Read the model definition and answer for the solid it produces. Units are mm, in the model's axes. A direction names the side the tool comes from. Coordinates: 2 decimals unless noted, no trailing zeros. Write each loop counter-clockwise with the first axis right and the second up, starting at its lowest first coordinate (ties: lowest second). Pieces come first, ordered by that corner, then holes. Notation, with made-up numbers: (51, -11) -> (62, -11) arc R22 cw to (62, 16) -> close; hole circle Ø6 at (-13.75, 65). An arc over 180 degrees is marked (long way). Answer as a JSON object with one key per item and string values. Group by question number.
(1) Find section A-A (y = -10). Give the vertices of the cut face in (x, z), then the cut area to 3 significant figures.
(2) Find section B-B (x = -7.5). Give the vertices of the cut face in (y, z).
(3) Straight lines are drawn through the part: L1, parallel to X at y = 13.14, z = -3.6; L2, parallel to Y at x = 13.25, z = -0.3; L3, parallel to X at y = 23.8, z = -2.5. For each, find the intervals that lie inside material, in ascending order.
(4) Which of the six approach directions +Z, -Z, +X, -X, +Y, -Y give full straight-line access (tool end or side, diameter ignored) to faces 4 (the face through (6, -29, -2)), 5 (the face through (-12.695, -24.458, -2.138)), 6 (the face through (-13, 27.5, -2)), 7 (the face through (-6, -29, -2)), 8 (the face through (11, 27.5, -2))?
(5) For a pull along Z with two mould halves and no side action, classify faces 1 (the face through (0, -13, 0)), 2 (the face through (-12, -21.5, -2)), 3 (the face through (13.106, -12.357, -2.535)) as +Z half, -Z half, draft (parallel to the pull), parting line (faces both ways), or undercut.
(6) Flat-ended cylindrical pins translate along their axes: P1, Ø1.3, axis at x = 12, z = -2, coming from the -Y side; P2, Ø1.7, axis at x = -12, z = -2.5, coming from the +Y side. Find the tip coordinate at first contact, or state that the pin passes through.
(7) Find section C-C (z = -0.75). Give the vertices of the cut face in (x, y).
Autodesk Inventor part; units mm, degrees
ref_plane "YZ Plane" through (0, 0, 0) normal (1, 0, 0) x (0, 1, 0)
ref_plane "XZ Plane" through (0, 0, 0) normal (0, 1, 0) x (-1, 0, 0)
ref_plane "XY Plane" through (0, 0, 0) normal (0, 0, 1) x (1, 0, 0)
sketch "Sketch1" plane through (0, 0, 0) normal (0, 0, 1) x (1, 0, 0)
  line L0 (15, 27.5) -> (-15, 27.5)
  line L1 (-15, 27.5) -> (-15, -27.5)
  line L2 (-15, -27.5) -> (15, -27.5)
  line L3 (15, -27.5) -> (15, 27.5)
  line L4 (15, 27.5) -> (-15, -27.5) construction
  line L5 (-15, 27.5) -> (15, -27.5) construction
  line L6 (13.14, 13.14) -> (-13.14, 13.14) construction
  line L7 (-13.14, 13.14) -> (-13.14, -13.14) construction
  line L8 (-13.14, -13.14) -> (13.14, -13.14) construction
  line L9 (13.14, -13.14) -> (13.14, 13.14) construction
  line L10 (13.14, 13.14) -> (-13.14, -13.14) construction
  line L11 (-13.14, 13.14) -> (13.14, -13.14) construction
  line L12 (15, 15) -> (-15, 15) construction
  line L13 (-15, 15) -> (-15, -15) construction
  line L14 (-15, -15) -> (15, -15) construction
  line L15 (15, -15) -> (15, 15) construction
  line L16 (15, 15) -> (-15, -15) construction
  line L17 (-15, 15) -> (15, -15) construction
  line L18 (0, 27.5) -> (0, -27.5) construction
  line L19 (15, 0) -> (-15, 0) construction
  line L20 (6, 27.5) -> (6, 30.5)
  line L21 (6, 30.5) -> (-6, 30.5)
  line L22 (-6, 30.5) -> (-6, 27.5)
  arc A0 (-9, 27.5) -> (-6, 27.5) centre (-7.5, 27.5) ccw
  line L23 (-15.1, -15.1) -> (15.1, 15.1) construction
  line L24 (15.1, -15.1) -> (-15.1, 15.1) construction
  line L25 (6, -27.5) -> (6, -30.5)
  line L26 (6, -30.5) -> (-6, -30.5)
  line L27 (-6, -30.5) -> (-6, -27.5)
  arc A1 (-6, -27.5) -> (-9, -27.5) centre (-7.5, -27.5) ccw
  line L28 (-12, 27.5) -> (-12, 21.5) construction
  line L29 (0, 30.5) -> (0, 27.5) construction
  line L30 (12, 27.5) -> (12, 21.5) construction
  arc A2 (6, 27.5) -> (9, 27.5) centre (7.5, 27.5) ccw
  line L31 (12, -27.5) -> (12, -21.5) construction
  arc A3 (9, -27.5) -> (6, -27.5) centre (7.5, -27.5) ccw
  circle A4 centre (0, 0) radius 12.5
  point P0 (13.14, -13.14)
  point P1 (-9, -27.5)
  point P2 (6, 28)
  point P3 (6, -27.5)
  point P4 (-6, -27.5)
  point P5 (-6, -27.5)
  point P6 (6, -27.5)
  point P7 (9, -27.5)
  dimension "d0" = 26.28
  dimension "d1" = 26.28
  dimension "d2" = 30
  dimension "d3" = 30
  dimension "d19" = 3
  dimension "d20" = 12
  dimension "d37" = 55
  dimension "d40" = 6
  dimension "d41" = 6
  dimension "d50" = 12.5
  dimension "d57" = 30
  dimension "d60" = 1.5
  dimension "d62" = 25
extrude "Extrusion1" add sketch "Sketch1" against normal blind 5 contours L3 L2 A3 A1 L1 L0 A0 A2 | L0 L22 L21 L20 | L25 L26 L27 L2 | A4
extrude "Extrusion2" cut sketch "Sketch1" against normal through all contours A4
hole "M2" at (13.14, 13.14, 0) at (-13.14, 13.14, 0) at (-13.14, -13.14, 0) at (13.14, -13.14, 0) direction (0, 0, -1) diameter 1.567 end through all
sketch "Sketch2" plane through (-15, 27.5, 0) normal (0, 1, 0) x (1, 0, 0)
  line L0 (3, 5) -> (3, 0)
  line L1 (30, 0) -> (0, 0)
  line L2 (27, 5) -> (27, 0)
  line L3 (24, 5) -> (30, 5)
  line L4 (0, 5) -> (6, 5)
  point P0 (15, 0)
  point P1 (6, 0)
  point P2 (3, 2.5)
  point P3 (3, 0)
  point P4 (27, 2.5)
  point P5 (27, 0)
hole "Side-M2" at (-12, 27.5, -2.5) at (12, 27.5, -2.5) direction (0, -1, 0) diameter 1.567 depth 6
mirror "Mirror1" about plane through (0, 0, 0) normal (0, 1, 0) of "Side-M2"
chamfer "C0.5" distance 0.5 angle 45 4 edges at (6, -30.5, -2.5) (-6, -30.5, -2.5) (6, 30.5, -2.5) (-6, 30.5, -2.5)
properties part number "HeadCameraMountFrame" material "Acetal Resin, Black"
Results below:
{
 "1": {"outline": "(-15, -5) -> (-7.5, -5) -> (-7.5, 0) -> (-15, 0) -> close; (7.5, -5) -> (15, -5) -> (15, 0) -> (7.5, 0) -> close", "area": "75.0 mm2"},
 "2": {"outline": "(-26, -5) -> (-10, -5) -> (-10, 0) -> (-26, 0) -> close; (10, -5) -> (26, -5) -> (26, 0) -> (10, 0) -> close"},
 "3": {"L1": "x = -15 to -13.92, -12.36 to 12.36, 13.92 to 15", "L2": "y = -27.5 to -13.92, -12.36 to 12.36, 13.92 to 27.5", "L3": "x = -15 to -12.78, -11.22 to 11.22, 12.78 to 15"},
 "4": {"face 4": "+Z, -Z, +X, -Y", "face 5": "-Y", "face 6": "+Z, -Z, -X, +Y", "face 7": "+Z, -Z, -X, -Y", "face 8": "+Z, -Z, +X, +Y"},
 "5": {"face 1": "+Z half", "face 2": "undercut", "face 3": "draft"},
 "6": {"P1": "stops at y = -27.5", "P2": "stops at y = 27.5"},
 "7": {"outline": "(-15, -27.5) -> (-9, -27.5) arc R1.5 cw to (-6, -27.5) -> (-6, -30) -> (-5.5, -30.5) -> (5.5, -30.5) -> (6, -30) -> (6, -27.5) arc R1.5 cw to (9, -27.5) -> (15, -27.5) -> (15, 27.5) -> (9, 27.5) arc R1.5 cw to (6, 27.5) -> (6, 30) -> (5.5, 30.5) -> (-5.5, 30.5) -> (-6, 30) -> (-6, 27.5) arc R1.5 cw to (-9, 27.5) -> (-15, 27.5) -> close; hole circle Ø1.57 at (-13.14, -13.14); hole circle Ø1.57 at (-13.14, 13.14); hole circle Ø25 at (0, 0); hole circle Ø1.57 at (13.14, -13.14); hole circle Ø1.57 at (13.14, 13.14)"}
}
